Can you work these out from the model? Positions are in its coordinate system, mm. Give positions to 0.01 mm unless a question says otherwise; leave off trailing zeros. Order: outer loops, then holes, each group sorted by start corner. A loop starts at its lowest first (then second) coordinate and runs counter-clockwise, first axis right, second up. Notation, with made-up numbers: (51.5, 65.25) - (100.5, 65.25) arc R20 ccw to (100.5, 83.25) - close; hole circle Ø2 at (-2.5, 34). An arc over 180 degrees is marked (long way). One line per question, with ' | ' between items.
Autodesk Inventor part; units mm, degrees
ref_plane "YZ Plane" through (0, 0, 0) normal (1, 0, 0) x (0, 1, 0)
ref_plane "XZ Plane" through (0, 0, 0) normal (0, 1, 0) x (-1, 0, 0)
ref_plane "XY Plane" through (0, 0, 0) normal (0, 0, 1) x (1, 0, 0)
sketch "Sketch1" plane through (0, 0, 0) normal (0, 1, 0) x (-1, 0, 0)
  line L0 (0, 0) -> (-30, 0)
  line L1 (-30, 0) -> (-30, 27)
  line L2 (-30, 27) -> (0, 27)
  line L3 (0, 27) -> (0, 0)
  dimension "d0" = 30
  dimension "d1" = 27
extrude "Extrusion1" add sketch "Sketch1" along normal blind 1
sketch "Sketch2" plane through (0, 1, 0) normal (0, 1, 0) x (1, 0, 0)
  line L0 (30, 0) -> (0, 0)
  line L1 (0, 0) -> (0, -27)
  line L2 (0, -27) -> (30, -27)
  line L3 (30, -27) -> (30, 0)
  line L4 (1.5, -25.5) -> (1.5, -1.5)
  line L5 (1.5, -1.5) -> (28.5, -1.5)
  line L6 (28.5, -1.5) -> (28.5, -25.5)
  line L7 (28.5, -25.5) -> (1.5, -25.5)
  circle A0 centre (1.5, -25.5) radius 1
  circle A1 centre (28.5, -25.5) radius 1
  circle A2 centre (1.5, -1.5) radius 1
  circle A3 centre (28.5, -1.5) radius 1
  dimension "d4" = 1.5
  dimension "d5" = 2
  dimension "d6" = 2
  dimension "d7" = 2
  dimension "d8" = 2
extrude "Extrusion2" cut sketch "Sketch2" against normal through all contours L7 A0 L4 | L4 A0 L7 | A2 L5 L4 | L4 L5 A2 | A1 L6 L7 | L7 L6 A1 | A3 L6 L5 | L5 L6 A3
properties part number "00_motordriver_pcb"
(1) If I drill on line 1 (X direction, y = 0.45, z = 25.5); line 2 (Z direction, x = 28.5, y = 0.4); line 3 (Z direction, x = 27.75, y = 0.5), over which ranges is the centre line in solid material (lowest first)?
Answer below:
line 1: 0 to 0.5, 2.5 to 27.5, 29.5 to 30 | line 2: 0 to 0.5, 2.5 to 24.5, 26.5 to 27 | line 3: 0 to 0.84, 2.16 to 24.84, 26.16 to 27
(2) Imagine slicing it at B-B (y = 0.3). List the corners of the cut face in (x, z) for me.
Answer below:
outline: (0, 0) - (30, 0) - (30, 27) - (0, 27) - close; hole circle Ø2 at (1.5, 1.5); hole circle Ø2 at (1.5, 25.5); hole circle Ø2 at (28.5, 1.5); hole circle Ø2 at (28.5, 25.5)
(3) Imagine slicing it at A-A (x = 1.5). List the corners of the cut face in (y, z) for me, and give its area (3 significant figures).
Answer below:
outline: (0, 0) - (1, 0) - (1, 0.5) - (0, 0.5) - close; (0, 2.5) - (1, 2.5) - (1, 24.5) - (0, 24.5) - close; (0, 26.5) - (1, 26.5) - (1, 27) - (0, 27) - close | area: 23.0 mm^2
(4) If we mould it in two halves opening along Z, with no side actions, what happens to faces 1 (the face through (15, 1, 14)), 2 (the face through (15.2, 0.5, 27)), 3 (the face through (1.283, 0.507, 2.476))? For each: released by +Z, released by -Z, zero draft, split by the parting line, or undercut.
Answer below:
face 1: zero draft | face 2: released by +Z | face 3: undercut
(5) Imagine slicing it at C-C (z = 1.5). List the corners of the cut face in (x, y) for me, and give its area (3 significant figures).
Answer below:
outline: (0, 0) - (0.5, 0) - (0.5, 1) - (0, 1) - close; (2.5, 0) - (27.5, 0) - (27.5, 1) - (2.5, 1) - close; (29.5, 0) - (30, 0) - (30, 1) - (29.5, 1) - close | area: 26.0 mm^2
